Here's how the part is built. I have some questions about the finished solid (model axes, mm). Face numbers are marked on the shaded views. A direction names the side the tool comes from. Coordinates: 2 decimals unless noted, no trailing zeros. Loops run counter-clockwise (first coordinate to the right, second up) from the corner with the lowest first, then second, coordinate; pieces in that order, holes last.
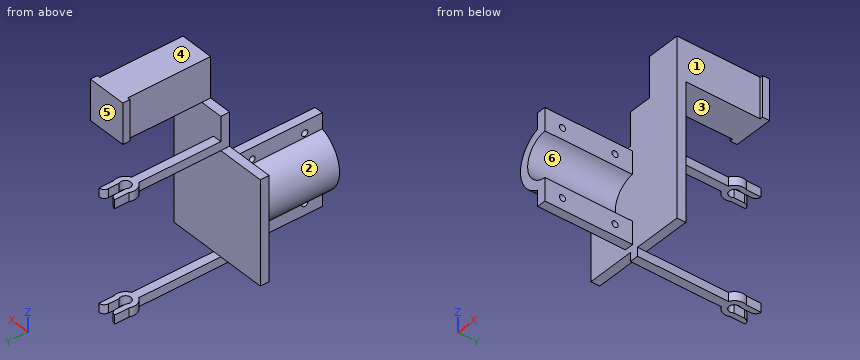
```python
from build123d import *

# Parameters (mm, degrees)
BOSS_EXTRUDE1_DEPTH = 5
SKETCH2_W           = 32.5
SKETCH2_H           = 5
BOSS_EXTRUDE2_DEPTH = 14
BOSS_EXTRUDE3_DEPTH = 23
SKETCH4_W           = 60
SKETCH4_H           = 5
BOSS_EXTRUDE4_DEPTH = 59
BOSS_EXTRUDE5_START = 5
BOSS_EXTRUDE5_DEPTH = 5
BOSS_EXTRUDE6_DEPTH = 50
SKETCH7_R           = 1.75
CUT_EXTRUDE1_DEPTH  = 130.133002576


with BuildPart() as part:
    # Sketch1 → Boss-Extrude1 (new body)
    with BuildSketch(Plane.XY):
        with BuildLine():
            Line((-2.5, -5.454356057), (-2.5, -57.315294131))
            Line((-2.5, -57.315294131), (30, -57.315294131))
            Line((30, -57.315294131), (30, -52.315294131))
            Line((30, -52.315294131), (2.5, -52.315294131))
            Line((2.5, -52.315294131), (2.5, -5.454356057))
            ThreePointArc((2.5, -5.454356057), (5.604867811, -2.141367979), (5.5, 2.397915762))
            Line((5.5, 2.397915762), (5.5, 10.658312395))
            ThreePointArc((5.5, 10.658312395), (3.378679656, 9.779632739), (2.5, 7.658312395))
            Line((2.5, 7.658312395), (2.5, 1.658312395))
            ThreePointArc((2.5, 1.658312395), (0, -3), (-2.5, 1.658312395))
            Line((-2.5, 1.658312395), (-2.5, 7.658312395))
            ThreePointArc((-2.5, 7.658312395), (-3.378679656, 9.779632739), (-5.5, 10.658312395))
            Line((-5.5, 10.658312395), (-5.5, 2.397915762))
            ThreePointArc((-5.5, 2.397915762), (-5.604867811, -2.141367979), (-2.5, -5.454356057))
        make_face()
    extrude(amount=BOSS_EXTRUDE1_DEPTH)

    # Sketch2 → Boss-Extrude2 (add)
    with BuildSketch(Plane.XY.offset(5)):
        with Locations((13.75, -54.815294131)):
            Rectangle(SKETCH2_W, SKETCH2_H)
    extrude(amount=BOSS_EXTRUDE2_DEPTH)

    # Sketch3 → Boss-Extrude3 (add)
    with BuildSketch(Plane.XY.offset(19)):
        Polygon((10.7, -57.315294131), (10.7, -9.9), (9.1, -9.9), (9.1, -5.9), (31.6, -5.9), (31.6, -9.9), (30, -9.9), (30, -57.315294131), align=None)
    extrude(amount=BOSS_EXTRUDE3_DEPTH)

    # Sketch4 → Boss-Extrude4 (add)
    with BuildSketch(Plane(origin=(0, 0, 0), x_dir=(-1, 0, 0), z_dir=(0, 0, -1))):
        with Locations((0, -54.815294131)):
            Rectangle(SKETCH4_W, SKETCH4_H)
    extrude(amount=BOSS_EXTRUDE4_DEPTH)

    # Sketch5 → Boss-Extrude5 (add)
    with BuildSketch(Plane(origin=(0, 0, -59), x_dir=(-1, 0, 0), z_dir=(0, 0, -1)).offset(BOSS_EXTRUDE5_START)):
        with BuildLine():
            Line((-2.5, -57.315294131), (2.5, -57.315294131))
            Line((2.5, -57.315294131), (2.5, -5.454356057))
            ThreePointArc((2.5, -5.454356057), (5.604867811, -2.141367979), (5.5, 2.397915762))
            Line((5.5, 2.397915762), (5.5, 10.658312395))
            ThreePointArc((5.5, 10.658312395), (3.378679656, 9.779632739), (2.5, 7.658312395))
            Line((2.5, 7.658312395), (2.5, 1.658312395))
            ThreePointArc((2.5, 1.658312395), (0, -3), (-2.5, 1.658312395))
            Line((-2.5, 1.658312395), (-2.5, 7.658312395))
            ThreePointArc((-2.5, 7.658312395), (-3.378679656, 9.779632739), (-5.5, 10.658312395))
            Line((-5.5, 10.658312395), (-5.5, 2.397915762))
            ThreePointArc((-5.5, 2.397915762), (-5.604867811, -2.141367979), (-2.5, -5.454356057))
            Line((-2.5, -5.454356057), (-2.5, -57.315294131))
        make_face()
    extrude(amount=-BOSS_EXTRUDE5_DEPTH)

    # Sketch6 → Boss-Extrude6 (add)
    with BuildSketch(Plane.XZ.offset(57.315294131)):
        with BuildLine():
            Line((-1, -3.529437252), (-1, -16.538518603))
            ThreePointArc((-1, -16.538518603), (-13, -29.5), (-1, -42.461481397))
            Line((-1, -42.461481397), (-1, -55.470562748))
            Line((-1, -55.470562748), (-6, -55.470562748))
            Line((-6, -55.470562748), (-6, -46.470562748))
            ThreePointArc((-6, -46.470562748), (-18, -29.5), (-6, -12.529437252))
            Line((-6, -12.529437252), (-6, -3.529437252))
            Line((-6, -3.529437252), (-1, -3.529437252))
        make_face()
    extrude(amount=BOSS_EXTRUDE6_DEPTH)

    # Sketch7 → Cut-Extrude1 (cut, through all)
    with BuildSketch(Plane(origin=(-1, 0, 0), x_dir=(0, 0, -1), z_dir=(1, 0, 0))):
        with Locations((10.033977927, -67.315294131)):
            Circle(SKETCH7_R)
        with Locations((10.033977927, -97.315294131)):
            Circle(SKETCH7_R)
        with Locations((48.966022073, -97.315294131)):
            Circle(SKETCH7_R)
        with Locations((48.966022073, -67.315294131)):
            Circle(SKETCH7_R)
    extrude(amount=-CUT_EXTRUDE1_DEPTH, mode=Mode.SUBTRACT)


solid = part.part
```
1. I want a section at B-B (z = -6). Please give me the cut outline in (x, y), then the cut area to 3 significant figures.
2. I need wall thicknesses on line 1 along X through (y, z) = (0, -61.65); line 2 along Z through (x, y) = (-1, -14); line 3 along Y through (x, z) = (-2.5, -27). Which ranges of each line are inside material? Lowest first, please.
3. I want a section at C-C (x = 26). Please give me the cut outline in (y, z), then the cut area to 3 significant figures.
4. On a 3-axis mill with a long thin cutter (end or side, diameter ignored), from which of +Z, -Z, +X, -X, +Y, -Y can I reach the whole of each face in a straight line? I mean the marked faces 1 and 2. Say none if no direction works.
5. We'd pull the mould along Z, two halves only. Please class the marked faces 3, 4, 5 and 6: +Z half, -Z half, draft (parallel to the pull), parting line (faces both ways), or undercut.
6. I want a section at D-D (y = -78.5). Please give me the cut outline in (x, z).
7. I want a section at A-A (y = 0). Please give me the cut outline in (x, z), then the cut area to 3 significant figures.
8. For pin 1 (13 mm diameter, centred on x = -1, y = -14.5, fed in from +Z); pin 2 (6 mm diameter, centred on x = 20, y = -12, fed in from -Z); pin 3 (1.3 mm diameter, centred on x = 30.5, z = 31.5, fed in from -Y), each with a flat end and sliding along its axis, tell me the tip position at first contact or that it passes through.
Response values:
1. outline: (-30, -57.32) - (-6, -57.32) - (-6, -107.32) - (-1, -107.32) - (-1, -57.32) - (30, -57.32) - (30, -52.32) - (-30, -52.32) - close
1. area: 550 mm2
2. line 1: x = -6 to -3, 3 to 6
2. line 2: z = -64 to -59, 0 to 5
2. line 3: y = -57.32 to -52.32
3. outline: (-57.32, -59) - (-52.32, -59) - (-52.32, 19) - (-5.9, 19) - (-5.9, 42) - (-57.32, 42) - close
3. area: 1,570 mm2
4. face 1: +Z, -Z, +X, -Y
4. face 2: -X, -Y
5. face 3: -Z half
5. face 4: +Z half
5. face 5: draft
5. face 6: undercut
6. outline: (-6, -55.47) - (-1, -55.47) - (-1, -42.46) arc R13 cw to (-1, -16.54) - (-1, -3.53) - (-6, -3.53) - (-6, -12.53) arc R18 ccw to (-6, -46.47) - close
7. outline: (-6, -64) - (-3, -64) - (-3, -59) - (-6, -59) - close; (-6, 0) - (-3, 0) - (-3, 5) - (-6, 5) - close; (3, -64) - (6, -64) - (6, -59) - (3, -59) - close; (3, 0) - (6, 0) - (6, 5) - (3, 5) - close
7. area: 60.0 mm2
8. pin 1: stops at z = 5
8. pin 2: stops at z = 19
8. pin 3: stops at y = -57.32
